Here's the drawing with two shaded views (mm, measured from the low corner). I have some questions. A direction names the side the tool comes from. Coordinates: 2 decimals unless noted, no trailing zeros. Loops run counter-clockwise (first coordinate to the right, second up) from the corner with the lowest first, then second, coordinate; pieces in that order, holes last. Notation, with made-up numbers: (-16.75, -27.5) -> (-0.75, -27.5) arc R25 cw to (-0.75, -1.5) -> close; hole circle Ø11 at (19, 67). An arc over 180 degrees is marked (long way). Answer as a JSON object with one key per item and string values. Group by question number.
1) I'm going to push flat-ended pins straight in: pin 1 (1 mm diameter, centred on x = 11, y = 12, fed in from +Z) (1 decimal); pin 2 (4 mm diameter, centred on x = 6.48, z = 8.56, fed in from +Y) (1 decimal); pin 3 (1 mm diameter, centred on x = 17, z = 6.5, fed in from -Y). Where does each tip first touch, or does it pass through?
2) I want a section at A-A (x = 2.5). Write out the boundary of the cut face in (y, z) (1 decimal).
3) I want a section at D-D (z = 10). Write out the boundary of the cut face in (x, y) (1 decimal).
4) I need wall thicknesses on probe 1 along Y at (x, z) = (20.5, 2) (1 decimal); probe 2 along X at (y, z) = (10.5, 2.25); probe 3 along X at (y, z) = (2, 7) (1 decimal). Which ranges of each line are inside material? Lowest first, please. Write a range as [from, to].
5) I want a section at C-C (y = 12). Write out the boundary of the cut face in (x, z) (1 decimal).
6) Which directions (+Z, -Z, +X, -X, +Y, -Y) give clear straight access to the entire face, cutting with the end or side of a thin tool? Please do the marked faces 1 and 2.
7) I want a section at B-B (z = 1.5). Write out the boundary of the cut face in (x, y) (1 decimal), then the cut area to 3 significant figures.
8) If we mould it in two halves opening along X, with no side actions, what happens to the marked faces 3, 4 and 5? For each: +X half, -X half, draft (parallel to the pull), parting line (faces both ways), or undercut.
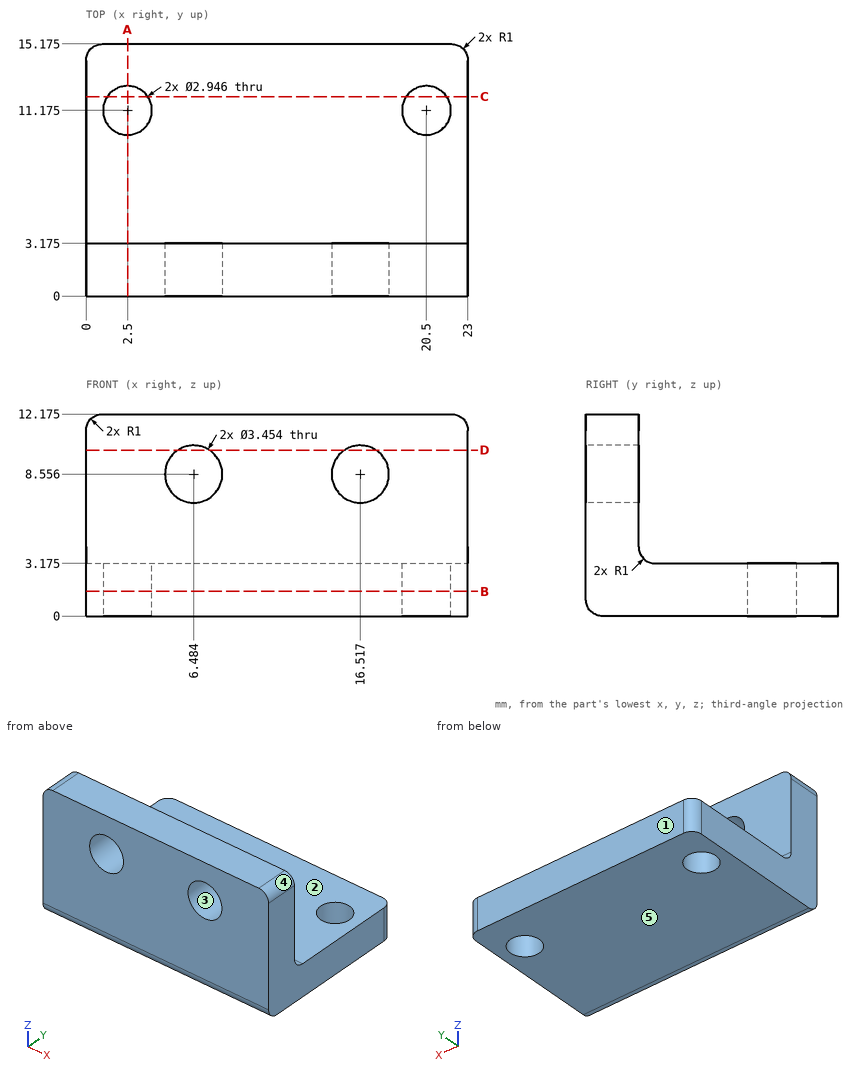
Determined:
{
 "1": {"pin 1": "z = 3.2", "pin 2": "y = 3.2", "pin 3": "y = 0"},
 "2": {"outline": "(0, 1) arc R1 ccw to (1, 0) -> (9.7, 0) -> (9.7, 3.2) -> (4.2, 3.2) arc R1 cw to (3.2, 4.2) -> (3.2, 12.2) -> (0, 12.2) -> close; (12.6, 0) -> (15.2, 0) -> (15.2, 3.2) -> (12.6, 3.2) -> close"},
 "3": {"outline": "(0, 0) -> (5.5, 0) -> (5.5, 3.2) -> (0, 3.2) -> close; (7.4, 0) -> (15.6, 0) -> (15.6, 3.2) -> (7.4, 3.2) -> close; (17.5, 0) -> (23, 0) -> (23, 3.2) -> (17.5, 3.2) -> close"},
 "4": {"probe 1": "[0, 9.7], [12.6, 15.2]", "probe 2": "[0, 1.19], [3.81, 19.19], [21.81, 23]", "probe 3": "[0, 5.7], [7.2, 15.8], [17.3, 23]"},
 "5": {"outline": "(0, 0) -> (1.3, 0) -> (1.3, 3.2) -> (0, 3.2) -> close; (3.7, 0) -> (19.3, 0) -> (19.3, 3.2) -> (3.7, 3.2) -> close; (21.7, 0) -> (23, 0) -> (23, 3.2) -> (21.7, 3.2) -> close"},
 "6": {"face 1": "+Z, -Z, +X, -X, +Y", "face 2": "+Z, +X, -X, +Y"},
 "7": {"outline": "(0, 0) -> (23, 0) -> (23, 14.2) arc R1 ccw to (22, 15.2) -> (1, 15.2) arc R1 ccw to (0, 14.2) -> close; hole circle Ø2.9 at (2.5, 11.2); hole circle Ø2.9 at (20.5, 11.2)", "area": "335 mm^2"},
 "8": {"face 3": "undercut", "face 4": "+X half", "face 5": "draft"}
}
